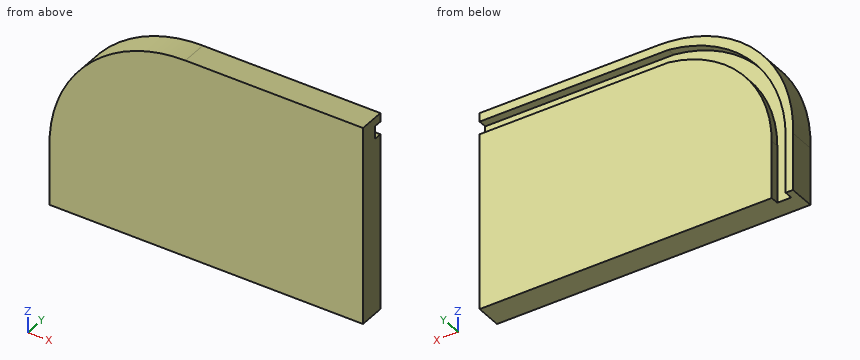
from build123d import *

# Parameters (mm, degrees)
F1_DEPTH = 25
F3_DEPTH = 8


with BuildPart() as f1:
    # F0 (on Front) → F1 (new body)
    with BuildSketch(Plane.XZ):
        with BuildLine():
            Line((-119.175632, 55), (-119.175632, 0))
            Line((-119.175632, 0), (180.824368, 0))
            Line((180.824368, 0), (180.824368, 190))
            Line((180.824368, 190), (10.824368, 190))
            ThreePointArc((10.824368, 190), (-82.883956, 150.145053), (-119.175632, 55))
        make_face()
    extrude(amount=F1_DEPTH)

    # F2 (on face) → F3 (cut)
    with BuildSketch(Plane(origin=(0, 0, 0), x_dir=(-1, 0, 0), z_dir=(0, 1, 0))):
        with BuildLine():
            Line((0, 181.738123), (-180.824368, 181.738123))
            Line((-180.824368, 181.738123), (-180.824368, 169.483781))
            Line((-180.824368, 169.483781), (0, 169.483781))
            ThreePointArc((0, 169.483781), (70.716626, 130.626464), (98.847926, 55))
            Line((98.847926, 55), (98.847926, 0))
            Line((98.847926, 0), (112.206072, 0))
            Line((112.206072, 0), (112.206072, 55))
            ThreePointArc((112.206072, 55), (80.123875, 139.635623), (0, 181.738123))
        make_face()
    extrude(amount=-F3_DEPTH, mode=Mode.SUBTRACT)


solid = f1.part
Work out the finished part from the listing and answer in its coordinate system (mm). Give positions to 0.01 mm unless a question says otherwise; leave off trailing zeros. Loops run counter-clockwise (first coordinate to the right, second up) from the corner with the lowest first, then second, coordinate; pieces in that order, holes last. Notation, with made-up numbers: (4.25, 61.25) - (45.25, 61.25) arc R7 ccw to (45.25, 74.25) - close; hole circle Ø4 at (-14.75, 32). An arc over 180 degrees is marked (long way). Answer in a Markdown table with one row per item.
(1) A flat-ended cylindrical pin translates along its axis: pin 1 Ø2.5 at (y, z) = (-5, 20.5) entering from -X. Find the tip coordinate at first contact, or state that the pin passes through.
Results list:
| item | result |
|---|---|
| pin 1 | stops at x = -119.18 |
(2) Section A-A (y = -4) is taken. Give the vertices of the cut face in (x, z), and give its area (3 significant figures).
Results list:
| item | result |
|---|---|
| outline | (-119.18, 0) - (-112.21, 0) - (-112.21, 55) arc R127.68 cw to (0, 181.74) - (180.82, 181.74) - (180.82, 190) - (10.82, 190) arc R130.09 ccw to (-119.18, 55) - close; (-98.85, 0) - (180.82, 0) - (180.82, 169.48) - (0, 169.48) arc R115.72 ccw to (-98.85, 55) - close |
| area | 48,200 mm² |
(3) Consider L1, parallel to X at y = -3.25, z = 19; L2, parallel to X at y = -3.5, z = 158.5; L3, parallel to Z at x = -64.5, y = -7.25. Determine where each line is inside the solid, lowest interval first. Write a range as [from, to].
Results list:
| item | result |
|---|---|
| L1 | x = [-119.18, -112.21], [-98.85, 180.82] |
| L2 | x = [-74.05, -59.29], [-34.89, 180.82] |
| L3 | z = [0, 137.28], [154.53, 165.97] |
(4) Section C-C (z = 119) is taken. Give the vertices of the cut face in (x, y).
Results list:
| item | result |
|---|---|
| outline | (-105.07, -25) - (180.82, -25) - (180.82, 0) - (-79.54, 0) - (-79.54, -8) - (-95.01, -8) - (-95.01, 0) - (-105.07, 0) - close |
(5) Section B-B (x = 146) is taken. Give the vertices of the cut face in (y, z).
Results list:
| item | result |
|---|---|
| outline | (-25, 0) - (0, 0) - (0, 169.48) - (-8, 169.48) - (-8, 181.74) - (0, 181.74) - (0, 190) - (-25, 190) - close |
